from build123d import *

# Parameters (mm, degrees)
F0_W     = 50
F0_H     = 50
F1_DEPTH = 3
F2_W     = 3
F2_H     = 25
F3_DEPTH = 3
F4_W     = 3
F4_H     = 25
F5_DEPTH = 3


with BuildPart() as f1:
    # F0 (on Front) → F1 (new body)
    with BuildSketch(Plane.XZ):
        with Locations((-35.504888, 0.668609)):
            Rectangle(F0_W, F0_H)
    extrude(amount=F1_DEPTH)

    # F2 (on face) → F3 (join)
    with BuildSketch(Plane.YZ.offset(-10.504888)):
        with Locations((-1.5, 1.168609)):
            Rectangle(F2_W, F2_H)
    extrude(amount=F3_DEPTH)

    # F4 (on face) → F5 (join)
    with BuildSketch(Plane(origin=(-60.504888, 0, 0), x_dir=(0, -1, 0), z_dir=(-1, 0, 0))):
        with Locations((1.5, 1.168609)):
            Rectangle(F4_W, F4_H)
    extrude(amount=F5_DEPTH)


solid = f1.part
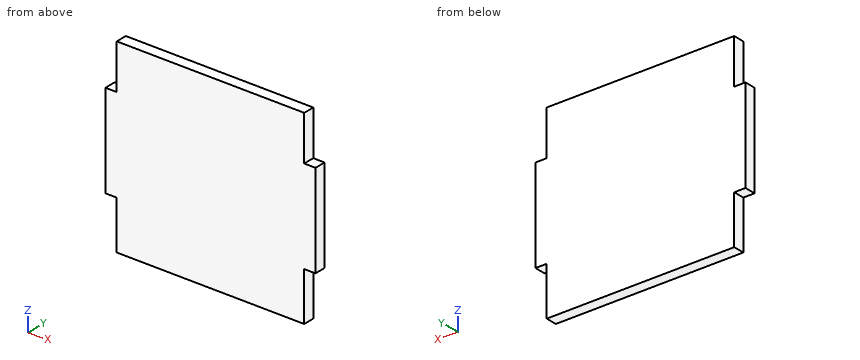
Geometry check sheet. Reference: the model listing, model coordinates, mm. Coordinates: 2 decimals unless noted, no trailing zeros. Write each loop counter-clockwise with the first axis right and the second up, starting at its lowest first coordinate (ties: lowest second). Pieces come first, ordered by that corner, then holes. Notation, with made-up numbers: (54, 23.25) -> (94, 23.25) arc R10 cw to (94, 35.25) -> close; hole circle Ø4 at (17.5, 66.25). An arc over 180 degrees is marked (long way). One line per question, with ' | ' between items.
1. Depth check by flat-ended pin: pin 1 Ø1.5 at (y, z) = (-1, -18) entering from +X; pin 2 Ø1.5 at (x, y) = (-8.5, -2) entering from -Z; pin 3 Ø0.9 at (y, z) = (-2, -19.5) entering from -X. Enter the tip coordinate at first touch or a pass-through.
Answers:
pin 1: stops at x = -10.5 | pin 2: stops at z = -11.33 | pin 3: stops at x = -60.5
2. Cross-section at B-B on z = 15. Record the cut outline in (x, y).
Answers:
outline: (-60.5, -3) -> (-10.5, -3) -> (-10.5, 0) -> (-60.5, 0) -> close
3. Cross-section at A-A on y = -2.2. Record the cut outline in (x, z).
Answers:
outline: (-63.5, -11.33) -> (-60.5, -11.33) -> (-60.5, -24.33) -> (-10.5, -24.33) -> (-10.5, -11.33) -> (-7.5, -11.33) -> (-7.5, 13.67) -> (-10.5, 13.67) -> (-10.5, 25.67) -> (-60.5, 25.67) -> (-60.5, 13.67) -> (-63.5, 13.67) -> close
4. Thickness scan on probe 1 along X at (y, z) = (-1.6, 14.5). Record the ranges inside material, lowest first. Write a range as from..to.
Answers:
probe 1: x = -60.5..-10.5
